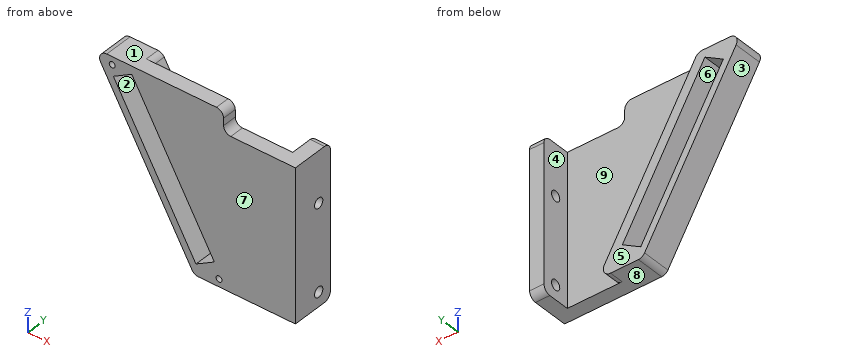
Autodesk Inventor part; units mm, degrees
ref_plane "YZ Plane" through (0, 0, 0) normal (1, 0, 0) x (0, 1, 0)
ref_plane "XZ Plane" through (0, 0, 0) normal (0, 1, 0) x (-1, 0, 0)
ref_plane "XY Plane" through (0, 0, 0) normal (0, 0, 1) x (1, 0, 0)
sketch "Sketch1" plane through (0, 0, 0) normal (0, 1, 0) x (-1, 0, 0)
  line L0 (47.3286, 48.1428) -> (-41.5714, 48.1428)
  line L1 (-41.5714, 48.1428) -> (-41.5714, -28.2969)
  line L2 (-41.5714, -28.2969) -> (3.1961, -28.2969)
  line L3 (47.3286, 48.1428) -> (3.1961, -28.2969)
  point P0 (0, 0)
  dimension "d0" = 60
  dimension "d1" = 88.265
  dimension "d2" = 88.9
extrude "Extrusion1" add sketch "Sketch1" along normal blind 6.35
sketch "Sketch2" plane through (41.5714, 0, 48.1428) normal (1, 0, 0) x (0, 0, -1)
  line L0 (0, 19.05) -> (76.4397, 19.05)
  line L1 (76.4397, 19.05) -> (76.4397, -12.7)
  line L2 (76.4397, -12.7) -> (0, -12.7)
  line L3 (0, -12.7) -> (0, 19.05)
  line L4 (0, 0) -> (76.4397, 0)
  line L5 (0, 6.35) -> (76.4397, 6.35)
  line L6 (0, 0) -> (0, 6.35)
  line L7 (76.4397, 0) -> (76.4397, 6.35)
  point P0 (48.1428, 0)
  dimension "d5" = 12.7
  dimension "d6" = 12.7
  dimension "d7" = 0
  dimension "d8" = 0
extrude "Extrusion2" add sketch "Sketch2" against normal blind 6.35 contours L0 L1 L5 L3 | L4 L1 L2 L3
sketch "Sketch3" plane through (0, 6.35, 0) normal (0, 1, 0) x (1, 0, 0)
  line L0 (-47.3286, -48.1428) -> (35.2214, -48.1428)
  line L1 (-3.1961, 28.2969) -> (-47.3286, -48.1428)
  line L2 (35.2214, 28.2969) -> (-3.1961, 28.2969)
  line L3 (-47.3286, -48.1428) -> (35.2214, -48.1428)
  line L4 (-47.3286, -48.1428) -> (-3.1961, 28.2969)
  line L5 (-3.1961, 28.2969) -> (16.4546, 28.2969)
  line L6 (35.2214, 28.2969) -> (-3.1961, 28.2969)
  line L7 (16.4546, 28.2969) -> (-27.6779, -48.1428)
  line L8 (-47.3286, -48.1428) -> (-27.6779, -48.1428)
  dimension "d13" = 17.018
extrude "Extrusion3" add sketch "Sketch3" along normal blind 6.35
sketch "Sketch4" plane through (0, 12.7, 0) normal (0, 1, 0) x (1, 0, 0)
  line L0 (-3.1961, 28.2969) -> (-47.3286, -48.1428)
  line L1 (-38.9235, -39.9348) -> (-2.411, 23.3067)
  line L2 (-2.411, 23.3067) -> (5.7279, 18.6077)
  line L3 (5.7279, 18.6077) -> (-30.7846, -44.6338)
  line L4 (-30.7846, -44.6338) -> (-38.9235, -39.9348)
  point P0 (0, 0)
  dimension "d16" = 9.398
  dimension "d17" = 3.175
  dimension "d18" = 73.025
extrude "Extrusion4" cut sketch "Sketch4" against normal blind 25.4
sketch "Sketch5" plane through (41.5714, 19.05, 48.1428) normal (1, 0, 0) x (0, 0, -1)
  line L0 (76.4397, -31.75) -> (0, -31.75)
  line L1 (76.4397, -31.75) -> (76.4397, 0)
  line L2 (0, 0) -> (76.4397, 0)
  point P0 (48.1428, -19.05)
  point P1 (70.0897, -6.35)
  point P2 (31.9897, -6.35)
  dimension "d22" = 0
  dimension "d23" = 6.35
  dimension "d24" = 38.1
  dimension "d48" = 6.35
hole "Hole1" at (41.5714, 12.7, -21.9469) at (41.5714, 12.7, 16.1531) direction (-1, 0, 0) diameter 4.4958 depth 25.4 tip angle 118.188
fillet "Fillet1" radius 3.175 1 edges at (-47.3286, 6.35, 48.1428)
fillet "Fillet2" radius 3.175 1 edges at (-3.1961, 6.35, -28.2969)
fillet "Fillet4" radius 3.175 6 edges at (38.3964, -12.7, -28.2969) (38.3964, -12.7, 48.1428) (38.3964, 19.05, -28.2969) (38.3964, 19.05, 48.1428) (16.4546, 9.525, -28.2969) (-27.6779, 9.525, 48.1428)
sketch "Sketch8" plane through (41.5714, -12.7, 44.9678) normal (1, 0, 0) x (0, 0, -1)
  line L0 (-49.5788, 45.5329) -> (6.35, 45.5329)
  line L1 (6.35, 45.5329) -> (6.35, -8.6732)
  line L2 (6.35, -8.6732) -> (-49.5788, -8.6732)
  line L3 (-49.5788, -8.6732) -> (-49.5788, 45.5329)
  line L4 (-3.175, 3.175) -> (-3.175, 28.575)
  point P0 (44.9678, 12.7)
  dimension "d41" = 9.525
extrude "Extrusion7" cut sketch "Sketch8" against normal blind 31.75
fillet "Fillet5" radius 3.175 1 edges at (9.8214, 3.175, 48.1428)
fillet "Fillet6" radius 3.175 2 edges at (38.3964, 19.05, 38.6178) (38.3964, -12.7, 38.6178)
fillet "Fillet7" radius 3.175 1 edges at (9.8214, 3.175, 38.6178)
sketch "Sketch10" plane through (41.5714, -9.525, -28.2969) normal (1, 0, 0) x (0, 0, -1)
  line L0 (-71.5248, -9.7742) -> (12.1423, -9.7742)
  line L1 (12.1423, -9.7742) -> (12.1423, 9.525)
  line L2 (12.1423, 9.525) -> (-71.5248, 9.525)
  line L3 (-71.5248, 9.525) -> (-71.5248, -9.7742)
  line L4 (0, 9.525) -> (-66.9147, 9.525)
  point P0 (-28.2969, 9.525)
  dimension "d49" = 0
extrude "Extrusion8" cut sketch "Sketch10" against normal blind 31.75
sketch "Sketch11" plane through (0, 0, 0) normal (0, -1, 0) x (1, 0, 0)
  point P0 (0, 0)
  point P1 (7.8072, -24.9207)
  point P2 (-39.4342, 44.6338)
hole "Hole2" at (7.8072, 0, -24.9207) at (-39.4342, 0, 44.6338) direction (0, 1, 0) diameter 2.6416 depth 10.9728 tip angle 118.188
properties part number "PhoneStandRight"
Design review of the part built by this model. Coordinates are the model's own, in mm. Face numbers are marked on the shaded views. A direction names the side the tool comes from. Coordinates: 2 decimals unless noted, no trailing zeros. Loops run counter-clockwise (first coordinate to the right, second up) from the corner with the lowest first, then second, coordinate; pieces in that order, holes last.
Item 1: Clearance check with flat-ended pins moving along their axes: pin 1 (8 mm diameter, centred on x = 4.5, z = 30, fed in from +Y); pin 2 (2.5 mm diameter, centred on y = 12.7, z = 16.15, fed in from -X); pin 3 (19.5 mm diameter, centred on x = -9.5, z = 26, fed in from +Y). State where each tip first meets the part, or that it passes through.
Completed:
pin 1: stops at y = 6.35
pin 2: stops at x = -29.58
pin 3: stops at y = 12.7
Item 2: Wall thickness on L1, parallel to Z at x = 39.75, y = 12.7; L2, parallel to X at y = 10.75, z = -16; L3, parallel to X at y = 6.5, z = -12: over which ranges is each line inside the solid? List them lowest first.
Completed:
L1: z = -28.3 to -24.19, -19.7 to 13.91, 18.4 to 38.62
L2: x = -10.3 to -6.63, 4.22 to 9.35, 35.22 to 41.57
L3: x = -12.61 to -8.94, 1.91 to 7.05, 35.22 to 41.57
Item 3: For the marked faces 5, 6, 7, 8 and 9, list the 3-axis set-ups (+Z, -Z, +X, -X, +Y, -Y) from which the entire face can be reached by the end or side of a thin tool; tool diameter is ignored.
Completed:
face 5: +Z, -Z, -X, +Y
face 6: +Y, -Y
face 7: +Z, -Z, +X, -X, -Y
face 8: -Z, +X, -X, +Y, -Y
face 9: +Z, +Y
Item 4: Add section D-D (z = 25). Write out the cut boundary in (x, y).
Completed:
outline: (-33.97, 0) - (-30.3, 0) - (-30.3, 12.7) - (-33.97, 12.7) - close; (-19.45, 0) - (41.57, 0) - (41.57, 19.05) - (35.22, 19.05) - (35.22, 6.35) - (-14.32, 6.35) - (-14.32, 12.7) - (-19.45, 12.7) - close
Item 5: Add section A-A (y = 8.75). Give the number of separate pieces and of enclosed holes in the cut face, and give its area (3 significant figures).
Completed:
separate pieces: 2
enclosed holes: 3
area: 1,210 mm2
Item 6: Draft analysis for pull direction Z (two halves, no side actions). For the marked faces 1, 2, 3 and 4, state which applies: pulls with the +Z half, pulls with the -Z half, needs draft (parallel to the pull), parting line crosses it, or undercut.
Completed:
face 1: pulls with the +Z half
face 2: undercut
face 3: pulls with the -Z half
face 4: needs draft
Item 7: Add section C-C (x = -34). Write out the cut boundary in (y, z).
Completed:
outline: (0, 25.06) - (12.7, 25.06) - (12.7, 31.41) - (0, 31.41) - close; (0, 42.78) - (12.7, 42.78) - (12.7, 48.14) - (0, 48.14) - close
Item 8: Add section B-B (x = 36.5). Write out the cut boundary in (y, z) (3 decimals), and give its area (3 significant figures).
Completed:
outline: (0, -28.297) - (15.875, -28.297) arc R3.175 ccw to (19.05, -25.122) - (19.05, 35.443) arc R3.175 ccw to (15.875, 38.618) - (0, 38.618) - close; hole circle Ø4.496 at (12.7, -21.947); hole circle Ø4.496 at (12.7, 16.153)
area: 1,240 mm2
